Answer from the drawing. Dimensions are ordinates in mm from the lowest x, y and z of the part. Coordinates: 2 decimals unless noted, no trailing zeros. Order: outer loops, then holes, each group sorted by start corner. A loop starts at its lowest first (then second) coordinate and runs counter-clockwise, first axis right, second up.
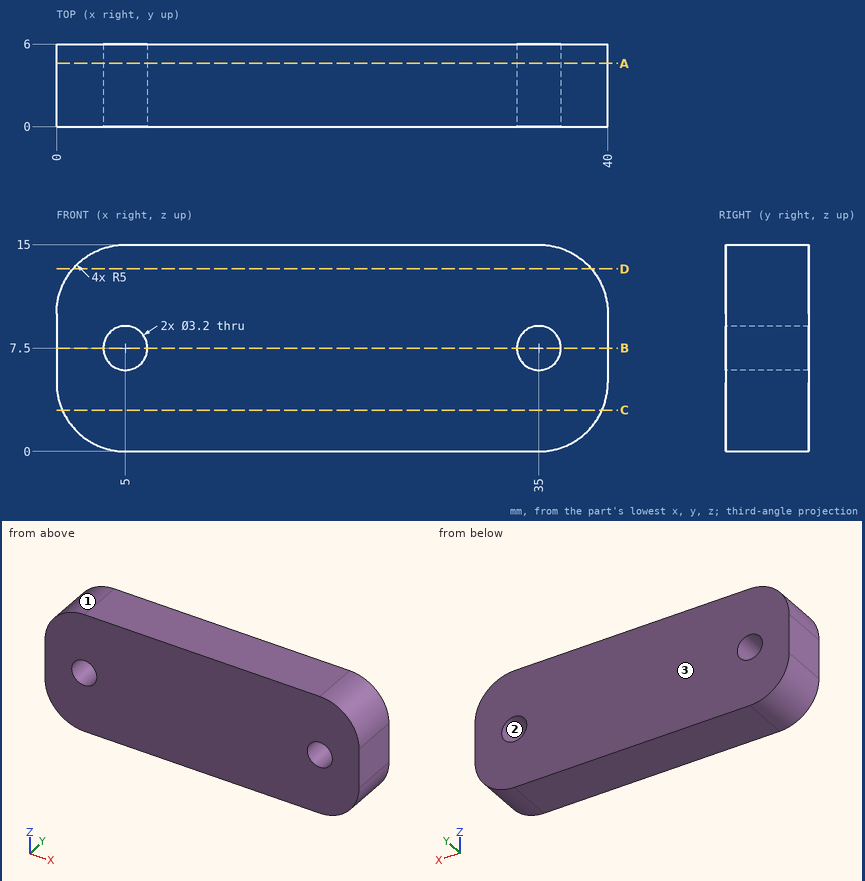
1. The part is cut by section C-C (z = 3). Determine the outline of the cut face in (x, y).
2. The part is cut by section A-A (y = 4.6). Determine the outline of the cut face in (x, z), plus the area to 3 significant figures.
3. The part is cut by section D-D (z = 13.25). Determine the outline of the cut face in (x, y), plus the area to 3 significant figures.
4. The part is cut by section B-B (z = 7.5). Determine the outline of the cut face in (x, y), plus the area to 3 significant figures.
5. The mould has two halves that part along X. Classify the marked faces 1, 2 and 3: released by +X, released by -X, zero draft, split by the parting line, or undercut.
6. A flat-ended cylindrical pin translates along its axis: pin 1 (2.5 mm diameter, centred on x = 35, z = 7.5, fed in from +Y). Find the tip coordinate at first contact, or state that the pin passes through.
7. Consider probe 1 along Z at (x, y) = (5, 2.6); probe 2 along X at (y, z) = (4.4, 8.75); probe 3 along X at (y, z) = (0.5, 6.5). Determine where each line is inside the solid, lowest interval first.
Worked out:
1. outline: (0.42, 0) - (39.58, 0) - (39.58, 6) - (0.42, 6) - close
2. outline: (0, 5) arc R5 ccw to (5, 0) - (35, 0) arc R5 ccw to (40, 5) - (40, 10) arc R5 ccw to (35, 15) - (5, 15) arc R5 ccw to (0, 10) - close; hole circle Ø3.2 at (5, 7.5); hole circle Ø3.2 at (35, 7.5)
2. area: 562 mm2
3. outline: (1.2, 0) - (38.8, 0) - (38.8, 6) - (1.2, 6) - close
3. area: 226 mm2
4. outline: (0, 0) - (3.4, 0) - (3.4, 6) - (0, 6) - close; (6.6, 0) - (33.4, 0) - (33.4, 6) - (6.6, 6) - close; (36.6, 0) - (40, 0) - (40, 6) - (36.6, 6) - close
4. area: 202 mm2
5. face 1: released by -X
5. face 2: undercut
5. face 3: zero draft
6. pin 1: passes through
7. probe 1: z = 0 to 5.9, 9.1 to 15
7. probe 2: x = 0 to 4, 6 to 34, 36 to 40
7. probe 3: x = 0 to 3.75, 6.25 to 33.75, 36.25 to 40
